Verification items for the finished model (mm, model axes). Round coordinates to 2 decimals unless told otherwise and drop trailing zeros. Write each loop counter-clockwise with the first axis right and the second up, starting at its lowest first coordinate (ties: lowest second). Pieces come first, ordered by that corner, then holes. Notation, with made-up numbers: (-16, 39.5) - (38, 39.5) arc R14 ccw to (38, 52.5) - close; hole circle Ø10 at (70.5, -37.5). An arc over 180 degrees is marked (long way). Write each question's results on one line, items separated by ' | '.
```python
from build123d import *

# Parameters (mm, degrees)
BOSS_EXTRUDE1_DEPTH = 1
SKETCH4_W           = 0.5
SKETCH4_H           = 4
CUT_EXTRUDE1_DEPTH  = 0.5


with BuildPart() as part:
    # Sketch3 → Boss-Extrude1 (new body)
    with BuildSketch(Plane(origin=(0, 0, 0), x_dir=(1, 0, 0), z_dir=(0, 1, 0))):
        Polygon((-2.031413613, 2.77486911), (-2.031413613, -1.22513089), (1.968586387, -1.22513089), (1.968586387, 2.77486911), (0.218586387, 2.77486911), (0.218586387, 6.77486911), (1.968586387, 6.77486911), (1.968586387, 10.77486911), (-2.031413613, 10.77486911), (-2.031413613, 6.77486911), (-0.281413613, 6.77486911), (-0.281413613, 2.77486911), align=None)
    extrude(amount=BOSS_EXTRUDE1_DEPTH)

    # Sketch4 → Cut-Extrude1 (cut)
    with BuildSketch(Plane(origin=(0, 1, 0), x_dir=(1, 0, 0), z_dir=(0, 1, 0))):
        with Locations((-0.031413613, 4.77486911)):
            Rectangle(SKETCH4_W, SKETCH4_H)
    extrude(amount=-CUT_EXTRUDE1_DEPTH, mode=Mode.SUBTRACT)


solid = part.part
```
(1) Thickness scan on L1, parallel to Z at x = -1.05, y = 0.4; L2, parallel to X at y = 0.4, z = -6.25. Record the ranges inside material, lowest first.
Answer:
L1: -10.77 to -6.77, -2.77 to 1.23 | L2: -0.28 to 0.22
(2) Mould release check, pull along Z, two halves, no side actions. Record for faces 1 (the flat face through (-0.1, 0.5, 1.225)), 2 (the flat face through (-0.1, 0.7, -6.775)), 3 (the flat face through (0, 1, -9)): released by +Z, released by -Z, zero draft, split by the parting line, or undercut.
Answer:
face 1: released by +Z | face 2: undercut | face 3: zero draft
(3) Section check C-C (y = 0.15). Record the cut outline in (x, z).
Answer:
outline: (-2.03, -10.77) - (1.97, -10.77) - (1.97, -6.77) - (0.22, -6.77) - (0.22, -2.77) - (1.97, -2.77) - (1.97, 1.23) - (-2.03, 1.23) - (-2.03, -2.77) - (-0.28, -2.77) - (-0.28, -6.77) - (-2.03, -6.77) - close
(4) Section check A-A (y = 0.85). Record the cut outline in (x, z).
Answer:
outline: (-2.03, -10.77) - (1.97, -10.77) - (1.97, -6.77) - (-2.03, -6.77) - close; (-2.03, -2.77) - (1.97, -2.77) - (1.97, 1.23) - (-2.03, 1.23) - close
(5) Section check B-B (x = 0.85). Record the cut outline in (y, z), plus the area to 3 significant figures.
Answer:
outline: (0, -10.77) - (1, -10.77) - (1, -6.77) - (0, -6.77) - close; (0, -2.77) - (1, -2.77) - (1, 1.23) - (0, 1.23) - close | area: 8.00 mm2
(6) Section check D-D (x = -0.1). Record the cut outline in (y, z).
Answer:
outline: (0, -10.77) - (1, -10.77) - (1, -6.77) - (0.5, -6.77) - (0.5, -2.77) - (1, -2.77) - (1, 1.23) - (0, 1.23) - close
